from build123d import *

# Parameters (mm, degrees)
ESQUISSE1_W      = 19.540548481
ESQUISSE1_H      = 47.905200599
ESQUISSE1_R      = 1
EXTRUSION1_DEPTH = 1
CHANFREIN1_SIZE  = 2


with BuildPart() as part:
    # Esquisse1 → Extrusion1 (new body)
    with BuildSketch(Plane.XY):
        with Locations((-42.09577401, -60.566266396)):
            Rectangle(ESQUISSE1_W, ESQUISSE1_H)
        with Locations((-37.268833007, -80.789072635)):
            Circle(ESQUISSE1_R, mode=Mode.SUBTRACT)
        with Locations((-47.471458714, -42.022391679)):
            Circle(ESQUISSE1_R, mode=Mode.SUBTRACT)
    extrude(amount=EXTRUSION1_DEPTH)

    # Chanfrein1
    chanfrein1_edges = [part.edges().sort_by_distance(p)[0] for p in [
        (-51.86604825, -36.613666097, 0.5),
        (-32.325499769, -36.613666097, 0.5),
        (-32.325499769, -84.518866696, 0.5),
        (-51.86604825, -84.518866696, 0.5),
    ]]
    chamfer(chanfrein1_edges, length=CHANFREIN1_SIZE)


solid = part.part
Part model, mm, in its own coordinate system. Give positions to 0.01 mm unless a question says otherwise; leave off trailing zeros. Write each loop counter-clockwise with the first axis right and the second up, starting at its lowest first coordinate (ties: lowest second). Pieces come first, ordered by that corner, then holes.
1) Cut at B-B on z = 0.45. Write the cut outline in (x, y), then the cut area to 3 significant figures.
Resolved:
outline: (-51.87, -82.52) - (-49.87, -84.52) - (-34.33, -84.52) - (-32.33, -82.52) - (-32.33, -38.61) - (-34.33, -36.61) - (-49.87, -36.61) - (-51.87, -38.61) - close; hole circle Ø2 at (-47.47, -42.02); hole circle Ø2 at (-37.27, -80.79)
area: 922 mm2
2) Probe L1, parallel to Y at x = -33.5, z = 0.4; L2, parallel to X at y = -83, z = 0.7; L3, parallel to Y at x = -50.25, z = 0.8. List the from-to ranges inside material, lowest first.
Resolved:
L1: y = -83.69 to -37.44
L2: x = -51.38 to -32.81
L3: y = -84.13 to -37
3) Two-plate mould, pull along X, no slides. Class faces 1 (the face through (-36.807, -81.676, 0.493)), 2 (the face through (-47.6, -41.03, 0.49)), 3 (the face through (-42.2, -36.614, 0.5)), 4 (the face through (-50.852, -83.533, 0.493)): released by +X, released by -X, zero draft, split by the parting line, or undercut.
Resolved:
face 1: undercut
face 2: undercut
face 3: zero draft
face 4: released by -X
4) Cut at A-A on x = -37.75. Write the cut outline in (y, z).
Resolved:
outline: (-84.52, 0) - (-81.67, 0) - (-81.67, 1) - (-84.52, 1) - close; (-79.91, 0) - (-36.61, 0) - (-36.61, 1) - (-79.91, 1) - close
